Could you check a few things on this model? Use its own coordinates, in mm. A direction names the side the tool comes from. Coordinates: 2 decimals unless noted, no trailing zeros. Write each loop counter-clockwise with the first axis right and the second up, starting at its lowest first coordinate (ties: lowest second). Pieces come first, ordered by that corner, then holes. Notation, with made-up numbers: (0.25, 15) - (23.25, 15) arc R36 cw to (23.25, 49) - close; hole circle Ø5 at (-35, -22). An arc over 180 degrees is marked (long way). Answer as a JSON object with one key per item and string values. Group by question number.
1) If we section it at C-C (y = -11.75): Write out the boundary of the cut face in (x, z).
2) On a 3-axis mill with a long thin cutter (end or side, diameter ignored), from which of +Z, -Z, +X, -X, +Y, -Y can I reach the whole of each face in a straight line? I mean faces 3 (the flat face through (13.5, -3.3, -5.6)), 4 (the cylindrical face through (7.89, -3.71, 9.82)), 5 (the cylindrical face through (7.888, -6.097, -11.412)). Say none if no direction works.
3) Will these pins go through, and if not, where does the flat tip stop? pin 1 Ø2 at (x, y) = (7.5, 5) entering from -Z; pin 2 Ø2.5 at (x, z) = (13.5, 1.5) entering from +Y; pin 3 Ø4 at (x, z) = (5.5, -11) entering from +Y.
4) We'd pull the mould along Z, two halves only. Please class faces 1 (the cylindrical face through (7.9, 12.1, -4.5)), 2 (the flat face through (16, 3, -6)): released by +Z, released by -Z, zero draft, split by the parting line, or undercut.
5) If we section it at B-B (y = 2.75): Write out the boundary of the cut face in (x, z).
6) If we section it at A-A (z = 0): Write out the boundary of the cut face in (x, y).
7) Please list where these lines run through material, in increasing order: line 1 along Y through (x, z) = (2.5, 0); line 2 along Z through (x, y) = (9.5, -13); line 3 along Z through (x, y) = (14.5, -10.75).
```python
from build123d import *

# Parameters (mm, degrees)
BASPROSKE_W        = 16
BASPROSKE_H        = 15
TOOTHCUT_DEPTH     = 27.570660511
TEETHCUTS_COUNT    = 13
TEETHCUTS_ANGLE    = 332.307692308
BORSKE_R           = 4
BORE_DEPTH         = 50.0000508
CUT_EXTRUDE1_DEPTH = 5


with BuildPart() as part:
    # BasProSke → Base-Revolve (revolve)
    with BuildSketch(Plane(origin=(0, 0, 0), x_dir=(1, 0, 0), z_dir=(0, 1, 0)), mode=Mode.PRIVATE) as base_revolve_sk:
        with Locations((8, 7.5)):
            Rectangle(BASPROSKE_W, BASPROSKE_H)
    revolve(base_revolve_sk.sketch.rotate(Axis((-10, 0, 0), (1, 0, 0)), 180), axis=Axis((-10, 0, 0), (1, 0, 0)))

    # TooCutSke → ToothCut (cut, through all)
    with BuildSketch(Plane(origin=(0, 0, 0), x_dir=(0, 0, -1), z_dir=(1, 0, 0))):
        with BuildLine():
            ThreePointArc((1.088245291, 10.442448141), (0, 10.499), (-1.088245291, 10.442448141))
            ThreePointArc((-1.088245291, 10.442448141), (-1.646045958, 12.816546547), (-3.224884568, 14.675243258))
            ThreePointArc((-3.224884568, 14.675243258), (0, 15.0254), (3.224884568, 14.675243258))
            ThreePointArc((3.224884568, 14.675243258), (1.646045958, 12.816546547), (1.088245291, 10.442448141))
        make_face()
    toothcut = extrude(amount=TOOTHCUT_DEPTH, mode=Mode.SUBTRACT)

    # TeethCuts: ToothCut ×13 about axis
    teethcuts_axis = Axis((-10, 0, 0), (1, 0, 0))
    for i in range(1, TEETHCUTS_COUNT):
        add(toothcut.rotate(teethcuts_axis, i * TEETHCUTS_ANGLE / (TEETHCUTS_COUNT - 1)), mode=Mode.SUBTRACT)

    # BorSke → Bore (cut, symmetric)
    with BuildSketch(Plane(origin=(0, 0, 0), x_dir=(0, 0, -1), z_dir=(1, 0, 0))):
        with Locations(Location((0, 0, 0), (0, 0, 180))):
            Circle(BORSKE_R)
    extrude(amount=BORE_DEPTH, both=True, mode=Mode.SUBTRACT)

    # Sketch1 → Cut-Extrude1 (cut)
    with BuildSketch(Plane(origin=(16, 0, 0), x_dir=(0, 0, -1), z_dir=(1, 0, 0))):
        Polygon((-3.75277675, 6.5), (-7.505553499, 0), (-3.75277675, -6.5), (3.75277675, -6.5), (7.505553499, 0), (3.75277675, 6.5), align=None)
    extrude(amount=-CUT_EXTRUDE1_DEPTH, mode=Mode.SUBTRACT)


solid = part.part
```
Here are the results:
{
 "1": {"outline": "(0, -7.43) - (16, -7.43) - (16, -4.43) - (0, -4.43) - close; (0, -1.6) - (16, -1.6) - (16, 1.6) - (0, 1.6) - close; (0, 4.43) - (16, 4.43) - (16, 7.43) - (0, 7.43) - close"},
 "2": {"face 3": "+X", "face 4": "+X, -X", "face 5": "-Z, +X, -X"},
 "3": {"pin 1": "stops at z = -14.16", "pin 2": "stops at y = 14.28", "pin 3": "stops at y = 11.49"},
 "4": {"face 1": "undercut", "face 2": "zero draft"},
 "5": {"outline": "(0, -11.74) - (16, -11.74) - (16, -5.92) - (11, -5.92) - (11, -2.9) - (0, -2.9) - close; (0, 2.9) - (11, 2.9) - (11, 5.92) - (16, 5.92) - (16, 11.74) - (0, 11.74) - close"},
 "6": {"outline": "(0, -15) - (16, -15) - (16, -6.5) - (11, -6.5) - (11, -4) - (0, -4) - close; (0, 4) - (11, 4) - (11, 6.5) - (16, 6.5) - (16, 10.5) - (0, 10.5) - close"},
 "7": {"line 1": "y = -15 to -4, 4 to 10.5", "line 2": "z = -7.34 to -5.74, -1.43 to 1.43, 5.74 to 7.34", "line 3": "z = -7.28 to -3.85, -1.52 to 1.52, 3.85 to 7.28"}
}
